from build123d import *

# Parameters (mm, degrees)
SKETCH1_R           = 7.9375
SKETCH1_R_2         = 0.9525
SKETCH1_R_3         = 0.254
BOSS_EXTRUDE1_DEPTH = 1.5875


with BuildPart() as part:
    # Sketch1 → Boss-Extrude1 (new body)
    with BuildSketch(Plane(origin=(0, 0, 0), x_dir=(1, 0, 0), z_dir=(0, 1, 0))):
        with Locations(Location((0, 0, 0), (0, 0, 270))):
            Circle(SKETCH1_R)
        with Locations(Location((-6.096, 0, 0), (0, 0, 270))):
            Circle(SKETCH1_R_2, mode=Mode.SUBTRACT)
        with Locations(Location((6.096, 0, 0), (0, 0, 270))):
            Circle(SKETCH1_R_2, mode=Mode.SUBTRACT)
        with Locations(Location((0, 2.54, 0), (0, 0, 270))):
            Circle(SKETCH1_R_3, mode=Mode.SUBTRACT)
        with Locations(Location((-2.54, 0, 0), (0, 0, 270))):
            Circle(SKETCH1_R_3, mode=Mode.SUBTRACT)
        with Locations(Location((0, -2.54, 0), (0, 0, 270))):
            Circle(SKETCH1_R_3, mode=Mode.SUBTRACT)
        with Locations(Location((2.54, 0, 0), (0, 0, 270))):
            Circle(SKETCH1_R_3, mode=Mode.SUBTRACT)
        Polygon((3.252691193, -2.545584412), (3.959797975, -3.252691193), (3.252691193, -3.959797975), (2.545584412, -3.252691193), align=None, mode=Mode.SUBTRACT)
    extrude(amount=BOSS_EXTRUDE1_DEPTH)


solid = part.part
Geometry: final body of the model. Coordinates: model frame, mm. Give positions to 0.01 mm unless a question says otherwise; leave off trailing zeros. Order: outer loops, then holes, each group sorted by start corner. A loop starts at its lowest first (then second) coordinate and runs counter-clockwise, first axis right, second up. Notation, with made-up numbers: (55, 41.25) - (75, 41.25) arc R23 ccw to (75, 59.25) - close; hole circle Ø9 at (-14.75, -28.75). An arc over 180 degrees is marked (long way). Use CSV: the item, a comma, the result in double quotes.
1. Section query A-A (z = 0). Output: boundary loops of the cut face in (x, y), plus the area to 3 significant figures.
Answers below:
outline,"(-7.94, 0) - (-7.05, 0) - (-7.05, 1.59) - (-7.94, 1.59) - close; (-5.14, 0) - (-2.79, 0) - (-2.79, 1.59) - (-5.14, 1.59) - close; (-2.29, 0) - (2.29, 0) - (2.29, 1.59) - (-2.29, 1.59) - close; (2.79, 0) - (5.14, 0) - (5.14, 1.59) - (2.79, 1.59) - close; (7.05, 0) - (7.94, 0) - (7.94, 1.59) - (7.05, 1.59) - close"
area,"17.5 mm2"
2. Contact query for a flat-ended pin moving along its axis: pin 1 (2.5 mm diameter, centred on x = 6.096, z = 0, fed in from +Y). Output: stop coordinate, or through.
Answers below:
pin 1,"y = 1.59"
3. Section query C-C (z = -2.54). Output: boundary loops of the cut face in (x, y), plus the area to 3 significant figures.
Answers below:
outline,"(-7.52, 0) - (-0.25, 0) - (-0.25, 1.59) - (-7.52, 1.59) - close; (0.25, 0) - (7.52, 0) - (7.52, 1.59) - (0.25, 1.59) - close"
area,"23.1 mm2"
4. Section query D-D (y = 1.35). Output: boundary loops of the cut face in (x, z) (1 decimal).
Answers below:
outline,"circle Ø15.9 at (0, 0); hole circle Ø1.9 at (-6.1, 0); hole circle Ø0.5 at (-2.5, 0); hole circle Ø0.5 at (0, -2.5); hole circle Ø0.5 at (0, 2.5); hole circle Ø0.5 at (2.5, 0); hole (2.5, 3.3) - (3.3, 2.5) - (4, 3.3) - (3.3, 4) - close; hole circle Ø1.9 at (6.1, 0)"
5. Material intervals for line 1 along X through (y, z) = (0.35, 0); line 2 along Z through (x, y) = (5.5, 1.15); line 3 along Z through (x, y) = (3, 0.7), sorted ascending. Write a range as from..to.
Answers below:
line 1,"-7.94..-7.05, -5.14..-2.79, -2.29..2.29, 2.79..5.14, 7.05..7.94"
line 2,"-5.72..-0.74, 0.74..5.72"
line 3,"-7.35..2.8, 3.71..7.35"
6. Mould query, pull axis X, two halves, no side actions, for faces 1 (the face through (0, 1.588, 0)), 2 (the face through (5.166, 0.783, -0.206)), 3 (the face through (-7.75, 0.78, -1.72)). Classes: +X half, -X half, draft (parallel to the pull), parting line (faces both ways), or undercut.
Answers below:
face 1,"draft"
face 2,"undercut"
face 3,"parting line"
7. Section query B-B (x = 0). Output: boundary loops of the cut face in (y, z).
Answers below:
outline,"(0, -7.94) - (1.59, -7.94) - (1.59, -2.79) - (0, -2.79) - close; (0, -2.29) - (1.59, -2.29) - (1.59, 2.29) - (0, 2.29) - close; (0, 2.79) - (1.59, 2.79) - (1.59, 7.94) - (0, 7.94) - close"
